CAD build for the part. Positions are in the model's coordinates, mm. A direction names the side the tool comes from. Give positions to 0.01 mm unless a question says otherwise; leave off trailing zeros. Write each loop counter-clockwise with the first axis right and the second up, starting at its lowest first coordinate (ties: lowest second). Pieces come first, ordered by that corner, then holes. Notation, with made-up numbers: (82, 27.5) - (135, 27.5) arc R19 cw to (135, 42.5) - close; hole circle Ø11 at (-38.5, -31.75). An arc over 180 degrees is marked (long way). Write item = value, one per line. Start each with the question number.
Autodesk Inventor part; units mm, degrees
ref_plane "Work Plane1" through (-95, 0, -119) normal (-1, 0, 0) x (0, 0, 1)
ref_plane "YZ Plane" through (0, 0, 0) normal (1, 0, 0) x (0, 1, 0)
ref_plane "XZ Plane" through (0, 0, 0) normal (0, 1, 0) x (-1, 0, 0)
sketch "Sketch1" plane through (0, 0, 0) normal (0, 1, 0) x (-1, 0, 0)
  line L0 (0, 0) -> (100, 0)
  line L1 (100, 0) -> (100, -119)
  line L2 (100, -119) -> (0, -119)
  line L3 (0, -119) -> (0, 0)
  dimension "d0" = 119
  dimension "d1" = 100
extrude "Extrusion1" add sketch "Sketch1" along normal blind 130
sketch "Sketch2" plane through (0, 0, -119) normal (0, 0, -1) x (-1, 0, 0)
  circle A0 centre (50, 65) radius 45
  line L0 (100, 0) -> (100, 130)
  line L1 (0, 0) -> (0, 130)
  line L2 (0, 0) -> (100, 0)
  line L3 (0, 130) -> (100, 130)
  circle A1 centre (50, 65) radius 36.5
  circle A2 centre (28.0236, 99.1226) radius 1.9
  line L4 (25.6342, 102.8326) -> (74.3658, 27.1674) construction
  line L5 (12.1674, 40.6342) -> (87.8326, 89.3658) construction
  dimension "d6" = 90
  dimension "d7" = 100
  dimension "d8" = 50
  dimension "d9" = 65
  dimension "d10" = 130
  dimension "d11" = 73
  dimension "d12" = 3.8
extrude "Extrusion2" cut sketch "Sketch2" against normal blind 8 contours A0 | A1 | A2
extrude "Extrusion3" cut sketch "Sketch2" against normal blind 18 contours A1
ref_plane "Work Plane1" through (-95, 0, -119) normal (-1, 0, 0) x (0, 0, 1)
sketch "Sketch3" plane through (-95, 0, -119) normal (-1, 0, 0) x (0, 0, 1)
  line L0 (18, 28.5) -> (18, 101.5)
  line L1 (119, 130) -> (119, 0)
  line L2 (119, 0) -> (0, 0)
  line L3 (0, 0) -> (0, 65)
  line L4 (8, 65) -> (0, 65)
  line L5 (0, 130) -> (119, 130)
  line L6 (0, 65) -> (0, 130)
  line L7 (114, 125) -> (18, 125)
  line L8 (18, 125) -> (18, 5)
  line L9 (18, 5) -> (114, 5)
  line L10 (114, 5) -> (114, 125)
  dimension "d16" = 5
  dimension "d17" = 5
  dimension "d18" = 5
extrude "Extrusion4" cut sketch "Sketch3" against normal blind 90 and the other way blind 90 contours L0 L8 L7 L10 L9
fillet "Fillet1" radius 5 8 edges at (-52.5, 5, -5) (-5, 5, -53) (-5, 65, -5) (-5, 125, -53) (-52.5, 125, -5) (-52.5, 5, -101) (-52.5, 125, -101) (-5, 65, -101)
sketch "Sketch8" plane through (-100, 0, -119) normal (-1, 0, 0) x (0, 0, 1)
  point P0 (119, 0)
sketch "Sketch10" plane through (-100, 0, -119) normal (-1, 0, 0) x (0, 0, 1)
  line L0 (0, 0) -> (119, 0)
  line L1 (119, 0) -> (119, 130)
  line L2 (0, 130) -> (119, 130)
  line L3 (0, 0) -> (0, 130)
extrude "Extrusion10" add sketch "Sketch10" along normal blind 5
sketch "Sketch12" plane through (0, 130, 0) normal (0, 1, 0) x (1, 0, 0)
  line L0 (0, 119) -> (-105, 119)
  line L1 (-105, 0) -> (-105, 119)
  line L2 (0, 0) -> (-105, 0)
  line L3 (0, 0) -> (0, 119)
  line L4 (-105, 0) -> (-100, 0)
  line L5 (-100, 0) -> (-100, 119)
  line L6 (-100, 119) -> (-105, 119)
  line L7 (-105, 119) -> (-105, 0)
  line L8 (-100, 20) -> (-105, 25)
  line L9 (-105, 40) -> (-100, 45)
  line L10 (-105, 94) -> (-100, 99)
  line L11 (-100, 74) -> (-105, 79)
  dimension "d82" = 119
  dimension "d86" = 5
  dimension "d87" = 45
  dimension "d88" = 45
  dimension "d90" = 45
  dimension "d91" = 45
  dimension "d92" = 20
  dimension "d93" = 25
  dimension "d94" = 20
  dimension "d95" = 25
extrude "Extrusion11" cut sketch "Sketch12" against normal blind 127 contours L5 L11 L1 L10 | L8 L1 L9 L5
fillet "Fillet2" radius 1 8 edges at (-105, 66.5, -25) (-100, 127.5, -20) (-105, 66.5, -40) (-100, 127.5, -45) (-105, 66.5, -79) (-100, 127.5, -74) (-105, 66.5, -94) (-100, 127, -99)
sketch "Sketch13" plane through (-10, 120, -5) normal (0, 0, -1) x (-1, 0, 0)
  line L0 (82.5, 0) -> (-2.5, 0)
  line L1 (-2.5, 0) -> (-2.5, -110)
  line L2 (-2.5, -110) -> (82.5, -110)
  line L3 (82.5, -110) -> (82.5, 0)
  line L4 (-5, 0) -> (-5, -110)
  line L5 (85, -110) -> (85, 0)
  circle A0 centre (78.5, -4.3) radius 1.8
  circle A1 centre (78.5, -4.3) radius 2.5
  line L6 (78.5, -4.3) -> (78.5, -140.0823) construction
  line L7 (78.5, -4.3) -> (-34.9987, -4.3) construction
  line L8 (1.5, 27.6777) -> (1.5, -220.2724) construction
  line L9 (-45.8754, -105.7) -> (99.6232, -105.7) construction
  line L10 (80, 5) -> (0, 5) construction
  line L11 (0, -115) -> (80, -115) construction
  circle A2 centre (78.5, -105.7) radius 1.8
  circle A3 centre (78.5, -105.7) radius 2.5
  circle A4 centre (1.5, -105.7) radius 1.8
  circle A5 centre (1.5, -105.7) radius 2.5
  circle A6 centre (1.5, -4.3) radius 1.8
  circle A7 centre (1.5, -4.3) radius 2.5
  point P0 (-10, -120)
  dimension "d97" = 85
  dimension "d98" = 110
  dimension "d99" = 90
  dimension "d100" = 2.5
  dimension "d101" = 4
  dimension "d102" = 4.3
  dimension "d103" = 3.6
  dimension "d104" = 5
  dimension "d105" = 4.3
  dimension "d107" = 120
  dimension "d108" = 5
  dimension "d109" = 4
  dimension "d110" = 3.6
  dimension "d111" = 5
  dimension "d112" = 3.6
  dimension "d113" = 5
  dimension "d114" = 3.6
  dimension "d115" = 5
extrude "Extrusion12" add sketch "Sketch13" along normal blind 3 contours A1 | A3 | A5 | A7
sketch "Sketch14" plane through (-105, 0, -119) normal (-1, 0, 0) x (0, 0, 1)
  line L0 (19.5, 52) -> (19.5, 34) construction
  line L1 (18, 52) -> (18, 34)
  line L2 (21, 34) -> (21, 52)
  arc A0 (21, 52) -> (18, 52) centre (19.5, 52) ccw
  arc A1 (18, 34) -> (21, 34) centre (19.5, 34) ccw
  line L3 (0, 130) -> (0, 0)
  line L4 (0, 0) -> (119, 0)
  point P0 (19.5, 43)
  dimension "d118" = 18
  dimension "d119" = 3
  dimension "d121" = 18
  dimension "d122" = 34
extrude "Extrusion13" cut sketch "Sketch14" against normal blind 20
sketch "Sketch15" plane through (-50, 65, -111) normal (0, 0, -1) x (-1, 0, 0)
  circle A0 centre (0, 0) radius 45 construction
  line L0 (31.8198, 31.8198) -> (-31.8198, -31.8198) construction
  line L1 (31.8198, -31.8198) -> (-31.8198, 31.8198) construction
  circle A1 centre (0, 0) radius 36.5 construction
  circle A2 centre (0, 0) radius 40.75 construction
  line L2 (0, -45) -> (0, 45) construction
  line L3 (-40, -60) -> (40, -60) construction
  circle A3 centre (28.8146, 28.8146) radius 1.8
  circle A4 centre (-28.8146, 28.8146) radius 1.8
  circle A5 centre (28.8146, -28.8146) radius 1.8
  circle A6 centre (-28.8146, -28.8146) radius 1.8
  point P0 (-50, -65)
  dimension "d125" = 45
  dimension "d126" = 73
  dimension "d129" = 90
  dimension "d130" = 4.25
  dimension "d131" = 3.6
  dimension "d135" = 3.6
  dimension "d136" = 3.6
  dimension "d137" = 3.6
extrude "Extrusion14" cut sketch "Sketch15" against normal blind 40
ref_plane "Work Plane2" through (-50, 0, -119) normal (-1, 0, 0) x (0, 0, 1)
split "Split1" plane through (-50, 0, -119) removes the side toward (-1, 0, 0)
sketch "Sketch18" plane through (-50, 0, -119) normal (-1, 0, 0) x (0, 0, 1)
  line L0 (8, 110) -> (0, 110)
  line L1 (8, 101.5) -> (8, 110)
  line L2 (18, 101.5) -> (8, 101.5)
  line L3 (18, 120) -> (18, 101.5)
  arc A0 (23, 125) -> (18, 120) centre (23, 120) ccw
  line L4 (109, 125) -> (23, 125)
  arc A1 (114, 120) -> (109, 125) centre (109, 120) ccw
  line L5 (114, 10) -> (114, 120)
  arc A2 (109, 5) -> (114, 10) centre (109, 10) ccw
  line L6 (23, 5) -> (109, 5)
  arc A3 (18, 10) -> (23, 5) centre (23, 10) ccw
  line L7 (18, 28.5) -> (18, 10)
  line L8 (8, 28.5) -> (18, 28.5)
  line L9 (8, 20) -> (8, 28.5)
  line L10 (0, 20) -> (8, 20)
  line L11 (0, 0) -> (0, 20)
  line L12 (119, 0) -> (0, 0)
  line L13 (119, 130) -> (119, 0)
  line L14 (0, 130) -> (119, 130)
  line L15 (0, 110) -> (0, 130)
  line L16 (117.7, 1.3) -> (1.3, 1.3)
  line L17 (1.3, 1.3) -> (1.3, 18.7)
  line L18 (1.3, 18.7) -> (9.3, 18.7)
  line L19 (9.3, 18.7) -> (9.3, 27.2)
  line L20 (9.3, 27.2) -> (16.7, 27.2)
  line L21 (16.7, 27.2) -> (16.7, 10)
  arc A4 (16.7, 10) -> (23, 3.7) centre (23, 10) ccw
  line L22 (23, 3.7) -> (109, 3.7)
  arc A5 (109, 3.7) -> (115.3, 10) centre (109, 10) ccw
  line L23 (115.3, 10) -> (115.3, 120)
  arc A6 (115.3, 120) -> (109, 126.3) centre (109, 120) ccw
  line L24 (109, 126.3) -> (23, 126.3)
  arc A7 (23, 126.3) -> (16.7, 120) centre (23, 120) ccw
  line L25 (16.7, 120) -> (16.7, 102.8)
  line L26 (16.7, 102.8) -> (9.3, 102.8)
  line L27 (9.3, 102.8) -> (9.3, 111.3)
  line L28 (9.3, 111.3) -> (1.3, 111.3)
  line L29 (1.3, 111.3) -> (1.3, 128.7)
  line L30 (1.3, 128.7) -> (117.7, 128.7)
  line L31 (117.7, 128.7) -> (117.7, 1.3)
  dimension "d140" = 1.3
equation "\"d8\" = 0.5 * d7"
equation "\"d9\" = 0.5 * d10"
equation "\"d100\" = -0.5 * d97 + 0.5 * d99"
equation "\"d108\" = -0.5 * d98 + 0.5 * d107"
equation "\"d130\" = -0.25 * d126 + 0.25 * d129"
equation "\"d135\" = d131"
equation "\"d136\" = d131"
equation "\"d137\" = d131"
properties part number "wooferBox"
1. Mould opens along Y. For faces 1 (the flat face through (-25, 130, -60)), 2 (the flat face through (-5, 66, -54)), 3 (the flat face through (-25, 64, 0)) say: +Y half, -Y half, draft (parallel to the pull), parting line (faces both ways), or undercut.
2. Cut at C-C (x = -37). Give the cut face in (y, z), then the cut area to 3 significant figures.
3. Cut at B-B (z = -25.5). Give the cut face in (x, y), then the cut area to 3 significant figures.
4. Pin check, flat tips, straight feed: pin 1 Ø8 at (x, y) = (-17, 49) entering from -Z; pin 2 Ø12 at (y, z) = (77.5, -69) entering from -X; pin 3 Ø22.5 at (x, y) = (-34, 81) entering from -Z. Stop position of each tip, or through.
5. Wall check: line 1 along Y through (x, z) = (-11, -84.5); line 2 along Z through (x, y) = (-12.5, 46); line 3 along Z through (x, y) = (-26, 117). Give the ranges that are in metal, low to high.
6. Cut at A-A (y = 65). Give the cut face in (x, z).
7. Tool access for faces 4 (the cylindrical face through (-22.2, 95.3, -106.1)), 5 (the cylindrical face through (-7, 6, -52)), 6 (the cylindrical face through (-11.266, 113.915, -6.479)): list every direction of +Z, -Z, +X, -X, +Y, -Y with a clear straight run to the whole face (end or side of a thin tool).
Output:
q1.face_1 = +Y half
q1.face_2 = undercut
q1.face_3 = draft
q2.outline = (0, -119) - (21.92, -119) - (21.92, -111) - (30.89, -111) - (30.89, -101) - (10, -101) arc R5 cw to (5, -96) - (5, -10) arc R5 cw to (10, -5) - (120, -5) arc R5 cw to (125, -10) - (125, -96) arc R5 cw to (120, -101) - (99.11, -101) - (99.11, -111) - (108.08, -111) - (108.08, -119) - (130, -119) - (130, 0) - (0, 0) - close
q2.area = 2,600 mm2
q3.outline = (-50, 0) - (0, 0) - (0, 130) - (-50, 130) - (-50, 125) - (-10, 125) arc R5 cw to (-5, 120) - (-5, 10) arc R5 cw to (-10, 5) - (-50, 5) - close
q3.area = 1,110 mm2
q4.pin_1 = -111
q4.pin_2 = -5
q4.pin_3 = -5
q5.line_1 = 0 to 5, 125 to 130
q5.line_2 = -111 to -101, -5 to 0
q5.line_3 = -119 to -101, -5 to 0
q6.outline = (-50, -5) - (-10, -5) arc R5 cw to (-5, -10) - (-5, -96) arc R5 cw to (-10, -101) - (-13.5, -101) - (-13.5, -111) - (-5, -111) - (-5, -119) - (0, -119) - (0, 0) - (-50, 0) - close
q7.face_4 = -Z
q7.face_5 = -X
q7.face_6 = none
